Part model, mm, in its own coordinate system. Give positions to 0.01 mm unless a question says otherwise; leave off trailing zeros. Order: outer loops, then holes, each group sorted by start corner. A loop starts at its lowest first (then second) coordinate and runs counter-clockwise, first axis right, second up.
1. Slice it at C-C on z = 0.45. List the corners of the cut face in (x, y) (1 decimal).
2. Slice it at B-B on x = 0. List the corners of the cut face in (y, z) (1 decimal), and give its area (3 significant figures).
3. Slice it at A-A on y = 0. List the corners of the cut face in (x, z) (1 decimal), and give its area (3 significant figures).
4. Probe line 1 (Y direction, x = -14, z = 1.2) (3 decimals); line 2 (X direction, y = 0.5, z = 1) (3 decimals); line 3 (Y direction, x = 0, z = 0.55) (3 decimals). List the from-to ranges inside material, lowest first.
5. Drop a flat-ended pin along its axis: pin 1 Ø0.8 at (x, z) = (-10.5, 1) entering from +Y (3 decimals). Give the stop position or say it passes through.
6. Slice it at D-D on x = 12.5. List the corners of the cut face in (y, z) (1 decimal).
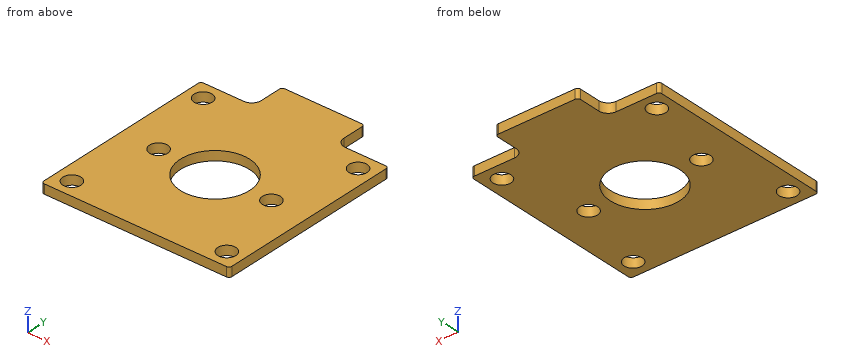
from build123d import *

# Parameters (mm, degrees)
BOSS_EXTRUDE1_DEPTH   = 1.5875
SKETCH2_R             = 5.842
CUT_EXTRUDE1_DEPTH    = 23.50669692
F_4_CLEARANCE_HOLE1_D = 3.048
SKETCH5_W             = 13.97
SKETCH5_H             = 11.43
BOSS_EXTRUDE2_DEPTH   = 1.5875
FILLET1_R             = 1.5875
FILLET2_R             = 0.508


with BuildPart() as part:
    # Sketch1 → Boss-Extrude1 (new body)
    with BuildSketch(Plane.XY):
        with BuildLine():
            Line((15.367, 15.875), (-15.367, 15.875))
            ThreePointArc((-15.367, 15.875), (-15.726210245, 15.726210245), (-15.875, 15.367))
            Line((-15.875, 15.367), (-15.875, -15.367))
            ThreePointArc((-15.875, -15.367), (-15.726210245, -15.726210245), (-15.367, -15.875))
            Line((-15.367, -15.875), (15.367, -15.875))
            ThreePointArc((15.367, -15.875), (15.726210245, -15.726210245), (15.875, -15.367))
            Line((15.875, -15.367), (15.875, 15.367))
            ThreePointArc((15.875, 15.367), (15.726210245, 15.726210245), (15.367, 15.875))
        make_face()
    extrude(amount=BOSS_EXTRUDE1_DEPTH)

    # Sketch2 → Cut-Extrude1 (cut, through all)
    with BuildSketch(Plane.XY.offset(1.5875)):
        Circle(SKETCH2_R)
    extrude(amount=-CUT_EXTRUDE1_DEPTH, mode=Mode.SUBTRACT)

    # #4 Clearance Hole1 (through all)
    with Locations(Plane.XY.offset(1.5875)):
        with Locations((-13.081, 13.081), (13.081, 13.081), (13.081, -13.081), (-13.081, -13.081), (-9.525, 0), (9.525, 0)):
            Hole(F_4_CLEARANCE_HOLE1_D / 2)

    # Sketch5 → Boss-Extrude2 (add, through all)
    with BuildSketch(Plane.XY.offset(1.5875)):
        with Locations((0, 15.875)):
            Rectangle(SKETCH5_W, SKETCH5_H)
    extrude(amount=-BOSS_EXTRUDE2_DEPTH)

    # Fillet1
    fillet1_edges = [part.edges().sort_by_distance(p)[0] for p in [
        (-6.985, 15.875, 0.79375),
        (6.985, 15.875, 0.79375),
    ]]
    fillet(fillet1_edges, radius=FILLET1_R)

    # Fillet2
    fillet2_edges = [part.edges().sort_by_distance(p)[0] for p in [
        (6.985, 21.59, 0.79375),
        (-6.985, 21.59, 0.79375),
    ]]
    fillet(fillet2_edges, radius=FILLET2_R)


solid = part.part
Data:
1. outline: (-15.9, -15.4) arc R0.5 ccw to (-15.4, -15.9) - (15.4, -15.9) arc R0.5 ccw to (15.9, -15.4) - (15.9, 15.4) arc R0.5 ccw to (15.4, 15.9) - (8.6, 15.9) arc R1.6 cw to (7, 17.5) - (7, 21.1) arc R0.5 ccw to (6.5, 21.6) - (-6.5, 21.6) arc R0.5 ccw to (-7, 21.1) - (-7, 17.5) arc R1.6 cw to (-8.6, 15.9) - (-15.4, 15.9) arc R0.5 ccw to (-15.9, 15.4) - close; hole circle Ø3 at (-13.1, -13.1); hole circle Ø3 at (-13.1, 13.1); hole circle Ø3 at (-9.5, 0); hole circle Ø11.7 at (0, 0); hole circle Ø3 at (9.5, 0); hole circle Ø3 at (13.1, -13.1); hole circle Ø3 at (13.1, 13.1)
2. outline: (-15.9, 0) - (-5.8, 0) - (-5.8, 1.6) - (-15.9, 1.6) - close; (5.8, 0) - (21.6, 0) - (21.6, 1.6) - (5.8, 1.6) - close
2. area: 40.9 mm2
3. outline: (-15.9, 0) - (-11, 0) - (-11, 1.6) - (-15.9, 1.6) - close; (-8, 0) - (-5.8, 0) - (-5.8, 1.6) - (-8, 1.6) - close; (5.8, 0) - (8, 0) - (8, 1.6) - (5.8, 1.6) - close; (11, 0) - (15.9, 0) - (15.9, 1.6) - (11, 1.6) - close
3. area: 22.2 mm2
4. line 1: y = -15.875 to -14.297, -11.865 to 11.865, 14.297 to 15.875
4. line 2: x = -15.875 to -10.965, -8.085 to -5.821, 5.821 to 8.085, 10.965 to 15.875
4. line 3: y = -15.875 to -5.842, 5.842 to 21.59
5. pin 1: stops at y = 15.875
6. outline: (-15.9, 0) - (-14.5, 0) - (-14.5, 1.6) - (-15.9, 1.6) - close; (-11.7, 0) - (11.7, 0) - (11.7, 1.6) - (-11.7, 1.6) - close; (14.5, 0) - (15.9, 0) - (15.9, 1.6) - (14.5, 1.6) - close
